Autodesk Inventor part; units mm, degrees
ref_plane "YZ Plane" through (0, 0, 0) normal (1, 0, 0) x (0, 1, 0)
ref_plane "XY Plane" through (0, 0, 0) normal (0, 0, 1) x (1, 0, 0)
sketch "Sketch1" plane through (0, 0, 0) normal (0, 0, 1) x (1, 0, 0)
  circle A0 centre (0, 0) radius 98.552
  circle A1 centre (0, 0) radius 101.6
  dimension "d0" = 197.104
  dimension "d1" = 203.2
extrude "Extrusion1" add sketch "Sketch1" along normal blind 200
ref_plane "Work Plane1" through (0, 101.6, 0) normal (0, 1, 0) x (-1, 0, 0)
ref_plane "Work Plane2" through (0, -101.6, 0) normal (0, 1, 0) x (-1, 0, 0)
sketch "Sketch7" plane through (0, -101.6, 0) normal (0, 1, 0) x (-1, 0, 0)
  circle A0 centre (0, 100) radius 19
  circle A1 centre (0, 100) radius 20
  line L0 (-101.6, 0) -> (101.6, 0)
  point P0 (0, 0)
  point P1 (20, 100)
  dimension "d11" = 40
  dimension "d12" = 38
  dimension "d13" = 100
extrude "Extrusion3" add sketch "Sketch7" along normal up to next
sketch "Sketch9" plane through (0, -101.6, 0) normal (0, 1, 0) x (-1, 0, 0)
  circle A0 centre (0, 100) radius 19
  circle A1 centre (0, 100) radius 20
  point P0 (0, 0)
  point P1 (20, 100)
  dimension "d16" = 40
  dimension "d17" = 38
extrude "Extrusion4" add sketch "Sketch9" against normal blind 50
sketch "Sketch10" plane through (0, -101.6, 0) normal (0, 1, 0) x (-1, 0, 0)
  circle A0 centre (0, 100) radius 19
  point P0 (0, 0)
  point P1 (20, 100)
extrude "Extrusion5" cut sketch "Sketch10" along normal through all
equation "\"BendRadius\" = Thickness"
equation "\"BendReliefWidth\" = Thickness"
equation "\"BendReliefDepth\" = 0.5 * Thickness"
equation "\"CornerReliefSize\" = 4 * Thickness"
equation "\"MinimumRemnant\" = 2 * Thickness"
equation "\"TransitionRadius\" = BendRadius"
equation "\"JacobiRadiusSize\" = Thickness"
equation "\"GapSize\" = Thickness"
properties part number "VacuumCylinder"
Geometry check sheet. Reference: the model listing, model coordinates, mm. Round coordinates to 2 decimals unless told otherwise and drop trailing zeros. Write each loop counter-clockwise with the first axis right and the second up, starting at its lowest first coordinate (ties: lowest second). Pieces come first, ordered by that corner, then holes. Notation, with made-up numbers: (36.5, -3.75) -> (54.5, -3.75) arc R21 cw to (54.5, 28.25) -> close; hole circle Ø8 at (-28.5, 22.5). An arc over 180 degrees is marked (long way). Put each result on its own line as item: value.
1) Cross-section at B-B, the plane x = -62. Enter the section's corners in (y, z).
Recorded:
outline: (-80.49, 0) -> (-76.61, 0) -> (-76.61, 200) -> (-80.49, 200) -> close; (76.61, 0) -> (80.49, 0) -> (80.49, 200) -> (76.61, 200) -> close
2) Release check for a two-part mould opening along Z. For faces 1 (the face through (-53.2, 83.3, 0)), 2 (the face through (-7, -151.6, 82)), 3 (the face through (14.004, 99.117, 87.159)), 4 (the face through (-53.2, 83.3, 200)) record: pulls with the +Z half, pulls with the -Z half, needs draft (parallel to the pull), parting line crosses it, or undercut.
Recorded:
face 1: pulls with the -Z half
face 2: needs draft
face 3: undercut
face 4: pulls with the +Z half
3) Cross-section at C-C, the plane z = 45. Enter the section's corners in (x, y), plus the area to 3 significant figures.
Recorded:
outline: circle Ø203.2 at (0, 0); hole circle Ø197.1 at (0, 0)
area: 1,920 mm2
4) Depth check by flat-ended pin: P1, Ø3, axis at y = -75, z = 133, coming from the +X side; P2, Ø6, axis at y = 73, z = 178, coming from the +X side; P3, Ø1, axis at x = -78, z = 104, coming from the -Y side. Enter the tip coordinate at first touch or a pass-through.
Recorded:
P1: stops at x = 70.14
P2: stops at x = 73.64
P3: stops at y = -65.7
5) Cross-section at D-D, the plane x = 14.5. Enter the section's corners in (y, z), plus the area to 3 significant figures.
Recorded:
outline: (-151.6, 86.23) -> (-100.56, 86.23) -> (-100.56, 0) -> (-97.48, 0) -> (-97.48, 87.72) -> (-151.6, 87.72) -> close; (-151.6, 112.28) -> (-97.48, 112.28) -> (-97.48, 200) -> (-100.56, 200) -> (-100.56, 113.77) -> (-151.6, 113.77) -> close; (97.48, 0) -> (100.56, 0) -> (100.56, 87.72) -> (97.48, 87.72) -> close; (97.48, 112.28) -> (100.56, 112.28) -> (100.56, 200) -> (97.48, 200) -> close
area: 1,230 mm2
6) Cross-section at A-A, the plane y = 0. Enter the section's corners in (x, z), plus the area to 3 significant figures.
Recorded:
outline: (-101.6, 0) -> (-98.55, 0) -> (-98.55, 200) -> (-101.6, 200) -> close; (98.55, 0) -> (101.6, 0) -> (101.6, 200) -> (98.55, 200) -> close
area: 1,220 mm2
7) Thickness scan on probe 1 along Y at (x, z) = (0, 78); probe 2 along X at (y, z) = (-140, 100). Record the ranges inside material, lowest first. Write a range as from..to.
Recorded:
probe 1: y = -101.6..-98.55, 98.55..101.6
probe 2: x = -20..-19, 19..20
